Autodesk Inventor part; units mm, degrees
ref_plane "YZ Plane" through (0, 0, 0) normal (1, 0, 0) x (0, 1, 0)
ref_plane "XZ Plane" through (0, 0, 0) normal (0, 1, 0) x (-1, 0, 0)
ref_plane "XY Plane" through (0, 0, 0) normal (0, 0, 1) x (1, 0, 0)
sketch "Esboço1" plane through (0, 0, 0) normal (0, 1, 0) x (-1, 0, 0)
  circle A0 centre (0, 0) radius 2.8
  dimension "d0" = 5.6
extrude "Extrusão1" add sketch "Esboço1" along normal blind 2.4
sketch "Esboço2" plane through (0, 0, 0) normal (1, 0, 0) x (0, 1, 0)
  line L0 (0, 0.9185) -> (1.2961, 0.9185)
  line L1 (1.2961, 0.9185) -> (1.2961, -0.9611)
  line L2 (1.2961, -0.9611) -> (0, -0.9611)
  line L3 (0, -0.9611) -> (0, 0.9185)
  point P0 (0, 0)
extrude "Extrusão2" cut sketch "Esboço2" along normal through all both and the other way through all
sketch "Esboço3" plane through (0, 2.4, 0) normal (0, 1, 0) x (1, 0, 0)
  circle A0 centre (0, 0) radius 2.8
  circle A1 centre (0, 0) radius 1.5
  dimension "d5" = 3
extrude "Extrusão3" add sketch "Esboço3" along normal blind 30 contours A1
thread "Rosca1"
properties part number "AA-Parafuso-M3-30"
Design review of the part built by this model. Coordinates are the model's own, in mm. A direction names the side the tool comes from. Give positions to 0.01 mm unless a question says otherwise; leave off trailing zeros. Order: outer loops, then holes, each group sorted by start corner. A loop starts at its lowest first (then second) coordinate and runs counter-clockwise, first axis right, second up.
1. Add section B-B, the plane x = -0.9. State the section outline as (y, z) points.
Solution:
outline: (0, -2.65) - (2.4, -2.65) - (2.4, -1.2) - (32.4, -1.2) - (32.4, 1.2) - (2.4, 1.2) - (2.4, 2.65) - (0, 2.65) - (0, 0.92) - (1.3, 0.92) - (1.3, -0.96) - (0, -0.96) - close
2. To check wall thickness, follow L1, parallel to Y at x = -1.8, z = 2.1; L2, parallel to Y at x = -0.4, z = 0.2; L3, parallel to X at y = 10.5, z = -0.05. State the ranges of each line that lie inside material, in increasing order.
Solution:
L1: y = 0 to 2.4
L2: y = 1.3 to 32.4
L3: x = -1.5 to 1.5
3. For pin 1 Ø1 at (x, y) = (-1, 0.5) entering from -Z (3 decimals); pin 2 Ø3 at (y, z) = (13.5, 1.5) entering from -X; pin 3 Ø3 at (x, y) = (0, 23.5) entering from -Z, all flat-tipped, find the tip position at first contact; note any pin that passes through.
Solution:
pin 1: stops at z = -2.755
pin 2: stops at x = -1.5
pin 3: stops at z = -1.5
4. Add section D-D, the plane x = -2.35. State the section outline as (y, z) points.
Solution:
outline: (0, -1.52) - (2.4, -1.52) - (2.4, 1.52) - (0, 1.52) - (0, 0.92) - (1.3, 0.92) - (1.3, -0.96) - (0, -0.96) - close
5. Add section A-A, the plane z = 0. State the section outline as (x, y) points, then the cut area to 3 significant figures.
Solution:
outline: (-2.8, 1.3) - (2.8, 1.3) - (2.8, 2.4) - (1.5, 2.4) - (1.5, 32.4) - (-1.5, 32.4) - (-1.5, 2.4) - (-2.8, 2.4) - close
area: 96.2 mm2
6. Add section C-C, the plane y = 27. State the section outline as (x, z) points.
Solution:
outline: circle Ø3 at (0, 0)
7. Tool access review of faces 1 (the flat face through (-1.2, 2.4, -1.2)), 2 (the flat face through (0, 1.296, 0)), 3 (the cylindrical face through (0.607, 1.183, 2.733)): name each direction out of +Z, -Z, +X, -X, +Y, -Y from which nothing blocks a thin tool from reaching the whole face with its end or side.
Solution:
face 1: +Y
face 2: +X, -X, -Y
face 3: +Y, -Y
